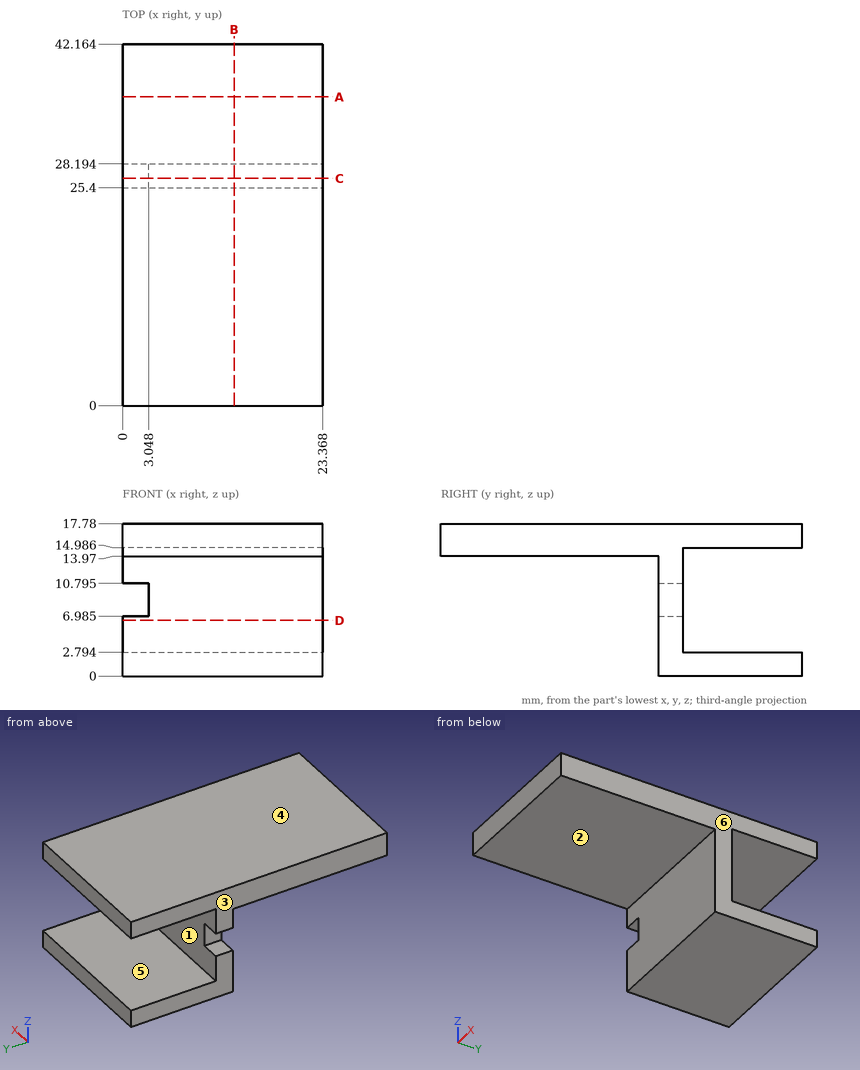
Check sheet for the drawn part. Datum: minimum x, y, z corner. Units: mm. A direction names the side the tool comes from. Round coordinates to 2 decimals unless told otherwise and drop trailing zeros. Order: outer loops, then holes, each group sorted by start corner. A loop starts at its lowest first (then second) coordinate and runs counter-clockwise, first axis right, second up.
(1) Scan lines: probe 1 along Z at (x, y) = (3.5, 38); probe 2 along Z at (x, y) = (15.75, 11); probe 3 along Z at (x, y) = (2.25, 28) (3 decimals). Record each from-to range of solid material in increasing order.
(2) Cross-section at B-B, the plane x = 13. Enter the section's corners in (y, z), and give its area (3 significant figures).
(3) Go/stop test with flat-tipped pins: P1, Ø4, axis at x = 8, z = 7.5, coming from the -Y side; P2, Ø2, axis at x = 19, y = 19.5, coming from the -Z side; P3, Ø6, axis at x = 17, z = 7, coming from the +Y side. Record where each tip stops, or that it passes through.
(4) Cross-section at C-C, the plane y = 26.5. Enter the section's corners in (x, z) (3 decimals), and give its area (3 significant figures).
(5) Cross-section at A-A, the plane y = 36. Enter the section's corners in (x, z), and give its area (3 significant figures).
(6) Draft check along Z on the marked faces 4, 5 and 6. Enter one of: pulls with the +Z half, pulls with the -Z half, needs draft (parallel to the pull), parting line crosses it, or undercut.
(7) Cross-section at D-D, the plane z = 6.5. Enter the section's corners in (x, y).
(8) Access from +Z, -Z, +X, -X, +Y, -Y to the whole of each face (thin tool, end or side, straight path). Record for the marked faces 1, 2 and 3.
Check sheet entries:
1. probe 1: z = 0 to 2.79, 14.99 to 17.78
1. probe 2: z = 13.97 to 17.78
1. probe 3: z = 0 to 6.985, 10.795 to 17.78
2. outline: (0, 13.97) - (25.4, 13.97) - (25.4, 0) - (42.16, 0) - (42.16, 2.79) - (28.19, 2.79) - (28.19, 14.99) - (42.16, 14.99) - (42.16, 17.78) - (0, 17.78) - close
2. area: 225 mm2
3. P1: stops at y = 25.4
3. P2: stops at z = 13.97
3. P3: stops at y = 28.19
4. outline: (0, 0) - (23.368, 0) - (23.368, 17.78) - (0, 17.78) - (0, 10.795) - (3.048, 10.795) - (3.048, 6.985) - (0, 6.985) - close
4. area: 404 mm2
5. outline: (0, 0) - (23.37, 0) - (23.37, 2.79) - (0, 2.79) - close; (0, 14.99) - (23.37, 14.99) - (23.37, 17.78) - (0, 17.78) - close
5. area: 131 mm2
6. face 4: pulls with the +Z half
6. face 5: undercut
6. face 6: needs draft
7. outline: (0, 25.4) - (23.37, 25.4) - (23.37, 28.19) - (0, 28.19) - close
8. face 1: +X, -X, +Y
8. face 2: -Z, +X, -X, -Y
8. face 3: +Z, -Z, -X, +Y, -Y
